```python
from build123d import *

# Parameters (mm, degrees)
F0_R        = 1.5
F0_R_2      = 1.3
F1_DEPTH    = 39.5
F2_DEPTH    = 1
F3_START    = -0.5
F3_DEPTH    = 0.5
F4_DEPTH    = 10
F5_R        = 1.3
F6_DEPTH    = 1
F7_START    = 0.5
F1_FACE_R   = 1.5
F1_FACE_R_2 = 1.3
F7_DEPTH    = 0.5
F8_SIZE     = 0.2
F9_SIZE     = 0.1


with BuildPart() as f1:
    # F0 (on Top) → F1 (new body)
    with BuildSketch(Plane.XY):
        Circle(F0_R)
        Circle(F0_R_2, mode=Mode.SUBTRACT)
        Circle(F0_R_2)
    extrude(amount=F1_DEPTH)

    # F0 (on Top) → F2 (join)
    with BuildSketch(Plane.XY):
        Circle(F0_R_2)
    extrude(amount=-F2_DEPTH)

    # F0 (on Top) → F3 (join)
    with BuildSketch(Plane.XY.offset(F3_START)):
        Circle(F0_R)
        Circle(F0_R_2, mode=Mode.SUBTRACT)
    extrude(amount=-F3_DEPTH)

    # F4 (add): a face of the model
    f4_faces = [f1.faces().sort_by_distance(p)[0] for p in [
        (0, 0, -1),
    ]]
    extrude(f4_faces, amount=F4_DEPTH)

    # F5 (on face) → F6 (join)
    with BuildSketch(Plane.XY.offset(39.5)):
        Circle(F5_R)
    extrude(amount=F6_DEPTH)

    # F1_face (on face) → F7 (join)
    with BuildSketch(Plane.XY.offset(39.5).offset(F7_START)):
        Circle(F1_FACE_R)
        Circle(F1_FACE_R_2, mode=Mode.SUBTRACT)
    extrude(amount=F7_DEPTH)

    # F8
    f8_edges = [f1.edges().sort_by_distance(p)[0] for p in [
        (-1.5, 0, 40.5),
        (-1.5, 0, -11),
    ]]
    chamfer(f8_edges, length=F8_SIZE)

    # F9
    f9_edges = [f1.edges().sort_by_distance(p)[0] for p in [
        (-1.5, 0, 39.5),
        (-1.5, 0, 40),
        (-1.5, 0, 0),
        (-1.5, 0, -0.5),
    ]]
    chamfer(f9_edges, length=F9_SIZE)


solid = f1.part
```
CAD build for the part. Positions are in the model's coordinates, mm. A direction names the side the tool comes from. Round coordinates to 2 decimals unless told otherwise and drop trailing zeros. Loops run counter-clockwise (first coordinate to the right, second up) from the corner with the lowest first, then second, coordinate; pieces in that order, holes last. Notation, with made-up numbers: M -26,49.25 L -21,49.25 A12 ccw -21,53.25 Z; hole C 82,8.25 d11. An arc over 180 degrees is marked long. Return JSON: item names as keys, results as strings. Group by question number.
(1) Drop a flat-ended pin along its axis: P1, Ø1.5, axis at x = 1, z = 19, coming from the +Y side. Give the stop position or say it passes through.
(2) Wall check: probe 1 along Z at (x, y) = (0.75, -1.25); probe 2 along Z at (x, y) = (-0.85, 1.1); probe 3 along X at (y, z) = (0.55, 8). Give the ranges that are in metal, low to high. Write a range as [from, to].
(3) Mould opens along Z. For faces 3 (the flat face through (0, 0, 40.5)), 4 (the cylindrical face through (-1.5, 0.07, -5.63)), 5 (the cylindrical face through (-0.17, 1.29, 39.75)) say: +Z half, -Z half, draft (parallel to the pull), parting line (faces both ways), or undercut.
(4) Saw through at A-A, the plane z = 18. List the corners of the cut face in (x, y).
(5) Tool access for faces 1 (the cylindrical face through (-0.17, 1.29, -0.25)), 2 (the cylindrical face through (-1.5, 0.07, 19.47)): list every direction of +Z, -Z, +X, -X, +Y, -Y with a clear straight run to the whole face (end or side of a thin tool).
Answer list:
{
 "1": {"P1": "y = 1.48"},
 "2": {"probe 1": "[-10.84, -0.56], [0.06, 39.44], [40.06, 40.34]", "probe 2": "[-10.91, -0.5], [0, 39.5], [40, 40.41]", "probe 3": "[-1.4, 1.4]"},
 "3": {"face 3": "+Z half", "face 4": "draft", "face 5": "undercut"},
 "4": {"outline": "C 0,0 d3"},
 "5": {"face 1": "none", "face 2": "+Z, -Z"}
}
